Source: CAD feature listing. Evaluate the final solid. Frame: model axes, mm. Round coordinates to 2 decimals unless told otherwise and drop trailing zeros. Loops run counter-clockwise (first coordinate to the right, second up) from the corner with the lowest first, then second, coordinate; pieces in that order, holes last. Notation, with made-up numbers: M 24,15 L 70,15 A6 cw 70,23 Z; hole C -8.75,63 d11. An arc over 180 degrees is marked long. Answer as a JSON object with one key per item and string values.
from build123d import *

# Parameters (mm, degrees)
SKETCH1_W           = 90
SKETCH1_H           = 250
BOSS_EXTRUDE1_DEPTH = 15
CHAMFER1_SIZE       = 15
FILLET1_R           = 10
SKETCH2_R           = 1.65
CUT_EXTRUDE1_DEPTH  = 267.129667643
SKETCH3_R           = 3
CUT_EXTRUDE2_DEPTH  = 3.3
SKETCH4_R           = 1.65
CUT_EXTRUDE3_DEPTH  = 267.129667643
CUT_EXTRUDE5_DEPTH  = 10


with BuildPart() as part:
    # Sketch1 → Boss-Extrude1 (new body)
    with BuildSketch(Plane(origin=(0, 0, 0), x_dir=(1, 0, 0), z_dir=(0, 1, 0))):
        with Locations((45, 125)):
            Rectangle(SKETCH1_W, SKETCH1_H)
    extrude(amount=BOSS_EXTRUDE1_DEPTH)

    # Chamfer1
    chamfer1_edges = [part.edges().sort_by_distance(p)[0] for p in [
        (45, 15, 0),
        (45, 15, -250),
    ]]
    chamfer(chamfer1_edges, length=CHAMFER1_SIZE - 0.0001)  # a hair under: the kernel refuses the full size

    # Fillet1
    fillet1_edges = [part.edges().sort_by_distance(p)[0] for p in [
        (0, 15, -125),
        (90, 15, -125),
    ]]
    fillet(fillet1_edges, radius=FILLET1_R)

    # Sketch2 → Cut-Extrude1 (cut, through all)
    with BuildSketch(Plane(origin=(0, 15, 0), x_dir=(1, 0, 0), z_dir=(0, 1, 0))):
        with Locations(Location((25, 30, 0), (0, 0, 270))):
            Circle(SKETCH2_R)
        with Locations(Location((65, 30, 0), (0, 0, 270))):
            Circle(SKETCH2_R)
        with Locations(Location((65, 220, 0), (0, 0, 90))):
            Circle(SKETCH2_R)
        with Locations(Location((25, 220, 0), (0, 0, 90))):
            Circle(SKETCH2_R)
    extrude(amount=-CUT_EXTRUDE1_DEPTH, mode=Mode.SUBTRACT)

    # Sketch3 → Cut-Extrude2 (cut)
    with BuildSketch(Plane(origin=(0, 15, 0), x_dir=(1, 0, 0), z_dir=(0, 1, 0))):
        with Locations(Location((25, 30, 0), (0, 0, 270))):
            Circle(SKETCH3_R)
        with Locations(Location((65, 30, 0), (0, 0, 270))):
            Circle(SKETCH3_R)
        with Locations(Location((65, 220, 0), (0, 0, 90))):
            Circle(SKETCH3_R)
        with Locations(Location((25, 220, 0), (0, 0, 90))):
            Circle(SKETCH3_R)
    extrude(amount=-CUT_EXTRUDE2_DEPTH, mode=Mode.SUBTRACT)

    # Sketch4 → Cut-Extrude3 (cut, through all)
    with BuildSketch(Plane(origin=(0, 15, 0), x_dir=(1, 0, 0), z_dir=(0, 1, 0))):
        with Locations(Location((45, 60, 0), (0, 0, 270))):
            Circle(SKETCH4_R)
        with Locations(Location((45, 129.4, 0), (0, 0, 270))):
            Circle(SKETCH4_R)
    extrude(amount=-CUT_EXTRUDE3_DEPTH, mode=Mode.SUBTRACT)

    # Sketch5 → Cut-Extrude5 (cut)
    with BuildSketch(Plane.XZ):
        Polygon((48.233161507, -60), (46.616580754, -57.2), (43.383419246, -57.2), (41.766838493, -60), (43.383419246, -62.8), (46.616580754, -62.8), align=None)
        Polygon((48.233161507, -129.4), (46.616580754, -126.6), (43.383419246, -126.6), (41.766838493, -129.4), (43.383419246, -132.2), (46.616580754, -132.2), align=None)
    extrude(amount=-CUT_EXTRUDE5_DEPTH, mode=Mode.SUBTRACT)


solid = part.part
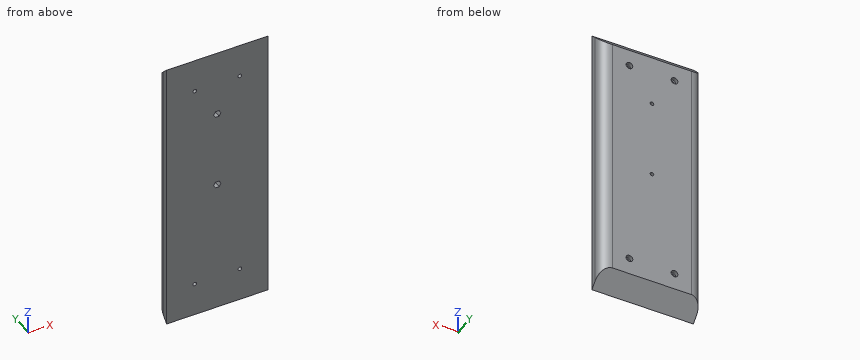
Item 1: Section A-A on z = -142. Return the cut outline in (x, y).
Answer sheet:
{"outline": "M 0,0 L 90,0 L 90,5 A10 ccw 80,15 L 10,15 A10 ccw 0,5 Z"}
Item 2: Contact query for flat-ended pins moving along their axis: pin 1 Ø4 at (x, z) = (25, -220) entering from +Y; pin 2 Ø8 at (x, y) = (31.5, 8.5) entering from -Z; pin 3 Ø1.5 at (y, z) = (10, -153) entering from -X. Output: stop coordinate, or through.
Answer sheet:
{"pin 1": "stops at y = 11.7", "pin 2": "stops at z = -245.5", "pin 3": "stops at x = 0.95"}
Item 3: Line query: probe 1 along Z at (x, y) = (46.5, 12.75); probe 2 along X at (y, z) = (13.2, -30); probe 3 along Z at (x, y) = (65, 6.75). Output: solid intervals per line, ascending. Write a range as from..to.
Answer sheet:
{"probe 1": "z = -237.25..-130.09, -128.71..-60.69, -59.31..-12.75", "probe 2": "x = 4.28..22, 28..62, 68..85.72", "probe 3": "z = -243.25..-221.65, -218.35..-31.65, -28.35..-6.75"}
